Model file for the job. Use its own axes, mm. Face numbers are marked on the shaded views. A direction names the side the tool comes from. Round coordinates to 2 decimals unless told otherwise and drop trailing zeros. Write each loop counter-clockwise with the first axis right and the second up, starting at its lowest first coordinate (ties: lowest second). Pieces come first, ordered by that corner, then holes. Notation, with made-up numbers: (13.5, -36) - (52.5, -36) arc R18 ccw to (52.5, -19) - close; hole circle Ø9 at (0.25, 64.5). An arc over 180 degrees is marked (long way). Answer as a JSON object with one key per item and string values. Group by question number.
from build123d import *

# Parameters (mm, degrees)
SKETCH1_W           = 52
SKETCH1_H           = 50
BOSS_EXTRUDE1_DEPTH = 4
SKETCH2_R           = 1.75
SKETCH2_R_2         = 11
CUT_EXTRUDE1_DEPTH  = 37.290494623
SKETCH3_W           = 4
SKETCH3_H           = 50
BOSS_EXTRUDE3_DEPTH = 48
BOSS_EXTRUDE4_START = -50
SKETCH5_W           = 20
SKETCH5_H           = 10
BOSS_EXTRUDE4_DEPTH = 50
SKETCH7_W           = 20
SKETCH7_H           = 44
CUT_EXTRUDE2_DEPTH  = 10
CUT_EXTRUDE3_DEPTH  = 77.681158051
CUT_EXTRUDE5_DEPTH  = 78.672388917
CUT_EXTRUDE6_DEPTH  = 61.041652209
CUT_EXTRUDE7_DEPTH  = 64.285069329


with BuildPart() as part:
    # Sketch1 → Boss-Extrude1 (new body)
    with BuildSketch(Plane(origin=(0, 0, 0), x_dir=(1, 0, 0), z_dir=(0, 1, 0))):
        Rectangle(SKETCH1_W, SKETCH1_H)
    extrude(amount=BOSS_EXTRUDE1_DEPTH)

    # Sketch2 → Cut-Extrude1 (cut, through all)
    with BuildSketch(Plane(origin=(0, 4, 0), x_dir=(1, 0, 0), z_dir=(0, 1, 0))):
        with Locations(Location((19, 15.5, 0), (0, 0, 270))):
            Circle(SKETCH2_R)
        with Locations(Location((-12, -15.5, 0), (0, 0, 90))):
            Circle(SKETCH2_R)
        with Locations(Location((19, -15.5, 0), (0, 0, 270))):
            Circle(SKETCH2_R)
        with Locations(Location((-12, 15.5, 0), (0, 0, 90))):
            Circle(SKETCH2_R)
        with Locations(Location((3.5, 0, 0), (0, 0, 270))):
            Circle(SKETCH2_R_2)
    extrude(amount=-CUT_EXTRUDE1_DEPTH, mode=Mode.SUBTRACT)

    # Sketch3 → Boss-Extrude3 (add)
    with BuildSketch(Plane(origin=(0, 4, 0), x_dir=(1, 0, 0), z_dir=(0, 1, 0))):
        with Locations((-24, 0)):
            Rectangle(SKETCH3_W, SKETCH3_H)
    extrude(amount=BOSS_EXTRUDE3_DEPTH)

    # Sketch5 → Boss-Extrude4 (add)
    with BuildSketch(Plane.XY.offset(25).offset(BOSS_EXTRUDE4_START)):
        with Locations((-12, 9)):
            Rectangle(SKETCH5_W, SKETCH5_H)
    extrude(amount=BOSS_EXTRUDE4_DEPTH)

    # Sketch7 → Cut-Extrude2 (cut)
    with BuildSketch(Plane(origin=(0, 14, 0), x_dir=(1, 0, 0), z_dir=(0, 1, 0))):
        with Locations((-12, 0)):
            Rectangle(SKETCH7_W, SKETCH7_H)
    extrude(amount=-CUT_EXTRUDE2_DEPTH, mode=Mode.SUBTRACT)

    # Sketch8 → Cut-Extrude3 (cut, through all)
    with BuildSketch(Plane.XY.offset(25)):
        Polygon((-22, 14), (-2, 4), (-2, 14), align=None)
    extrude(amount=-CUT_EXTRUDE3_DEPTH, mode=Mode.SUBTRACT)

    # Sketch9 → Cut-Extrude5 (cut, through all)
    with BuildSketch(Plane.ZY.offset(26)):
        with BuildLine():
            Line((-13.75, 47.315114044), (-13.75, 8.684885956))
            ThreePointArc((-13.75, 8.684885956), (-15.5, 6.934885956), (-17.25, 8.684885956))
            Line((-17.25, 8.684885956), (-17.25, 47.315114044))
            ThreePointArc((-17.25, 47.315114044), (-15.5, 49.065114044), (-13.75, 47.315114044))
        make_face()
        with BuildLine():
            Line((17.25, 47.315114044), (17.25, 8.684885956))
            ThreePointArc((17.25, 8.684885956), (15.5, 6.934885956), (13.75, 8.684885956))
            Line((13.75, 8.684885956), (13.75, 47.315114044))
            ThreePointArc((13.75, 47.315114044), (15.5, 49.065114044), (17.25, 47.315114044))
        make_face()
    extrude(amount=-CUT_EXTRUDE5_DEPTH, mode=Mode.SUBTRACT)

    # Sketch11 → Cut-Extrude6 (cut, through all)
    with BuildSketch(Plane(origin=(0, 4, 0), x_dir=(1, 0, 0), z_dir=(0, 1, 0))):
        with BuildLine():
            Line((-16.2, 17.25), (-7.8, 17.25))
            ThreePointArc((-7.8, 17.25), (-6.05, 15.5), (-7.8, 13.75))
            Line((-7.8, 13.75), (-16.2, 13.75))
            ThreePointArc((-16.2, 13.75), (-17.95, 15.5), (-16.2, 17.25))
        make_face()
        with BuildLine():
            Line((-16.2, -17.25), (-7.8, -17.25))
            ThreePointArc((-7.8, -17.25), (-6.05, -15.5), (-7.8, -13.75))
            Line((-7.8, -13.75), (-16.2, -13.75))
            ThreePointArc((-16.2, -13.75), (-17.95, -15.5), (-16.2, -17.25))
        make_face()
        with BuildLine():
            Line((23.2, 13.75), (14.8, 13.75))
            ThreePointArc((14.8, 13.75), (13.05, 15.5), (14.8, 17.25))
            Line((14.8, 17.25), (23.2, 17.25))
            ThreePointArc((23.2, 17.25), (24.95, 15.5), (23.2, 13.75))
        make_face()
        with BuildLine():
            Line((23.2, -13.75), (14.8, -13.75))
            ThreePointArc((14.8, -13.75), (13.05, -15.5), (14.8, -17.25))
            Line((14.8, -17.25), (23.2, -17.25))
            ThreePointArc((23.2, -17.25), (24.95, -15.5), (23.2, -13.75))
        make_face()
    extrude(amount=-CUT_EXTRUDE6_DEPTH, mode=Mode.SUBTRACT)

    # Sketch12 → Cut-Extrude7 (cut, through all)
    with BuildSketch(Plane.XZ):
        with BuildLine():
            Line((3.5, -11), (-4.5, -11))
            ThreePointArc((-4.5, -11), (-15.5, 0), (-4.5, 11))
            Line((-4.5, 11), (3.5, 11))
            ThreePointArc((3.5, 11), (14.5, 0), (3.5, -11))
        make_face()
    extrude(amount=-CUT_EXTRUDE7_DEPTH, mode=Mode.SUBTRACT)


solid = part.part
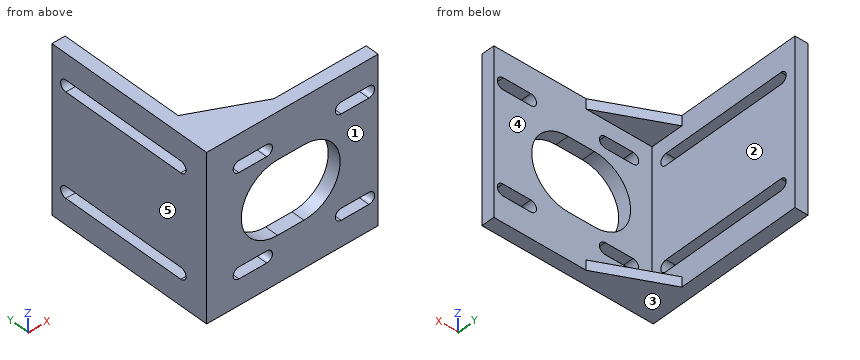
(1) Pull direction Z, two halves, no side cores. Call the marked faces 3, 4 and 5: pulls with the +Z half, pulls with the -Z half, needs draft (parallel to the pull), parting line crosses it, or undercut.
(2) Slice it at D-D (y = 5). Write the cut outline in (x, z).
(3) Slice it at B-B (y = 32). Write the cut outline in (x, z).
(4) Slice it at A-A (z = 0). Write the cut outline in (x, y).
(5) 3-axis set-ups, long thin cutter, end or side, ignore diameter. For the marked faces 1 and 2: which of +Z, -Z, +X, -X, +Y, -Y reach the whole face in a straight line?
(6) Slice it at C-C (z = 15.5). Write the cut outline in (x, y), then the cut area to 3 significant figures.
(7) Drill centre lines: line 1 (Z direction, x = -22.5, y = 7.5); line 2 (X direction, y = 6, z = 10); line 3 (Y direction, x = 22, z = -13.5). Where is each one in solid material? Low to high. Write a range as from..to.
(8) Flat gauge pins, fed straight in: pin 1 (5 mm diameter, centred on x = 16, z = 10, fed in from +Y); pin 2 (24 mm diameter, centred on y = 37.5, z = 1, fed in from +X). Where does each tip first touch, or does it go through?
Answer:
{
 "1": {"face 3": "pulls with the -Z half", "face 4": "undercut", "face 5": "needs draft"},
 "2": {"outline": "(-26, -25) - (-4, -25) - (-4, -22) - (-22, -22) - (-22, 22) - (-4, 22) - (-4, 25) - (-26, 25) - close"},
 "3": {"outline": "(-26, -25) - (-22, -25) - (-22, -17.25) - (-26, -17.25) - close; (-26, -13.75) - (-22, -13.75) - (-22, 13.75) - (-26, 13.75) - close; (-26, 17.25) - (-22, 17.25) - (-22, 25) - (-26, 25) - close"},
 "4": {"outline": "(-26, 0) - (-15.5, 0) - (-15.5, 4) - (-22, 4) - (-22, 52) - (-26, 52) - close; (14.5, 0) - (26, 0) - (26, 4) - (14.5, 4) - close"},
 "5": {"face 1": "+Z, -Z, +X, -X, -Y", "face 2": "+X, +Y"},
 "6": {"outline": "(-26, 0) - (-17.95, 0) - (-17.95, 4) - (-22, 4) - (-22, 6.93) - (-26, 6.93) - close; (-26, 49.07) - (-22, 49.07) - (-22, 52) - (-26, 52) - close; (-6.05, 0) - (13.05, 0) - (13.05, 4) - (-6.05, 4) - close; (24.95, 0) - (26, 0) - (26, 4) - (24.95, 4) - close", "area": "136 mm²"},
 "7": {"line 1": "-25..-16.79, -14.21..14.21, 16.79..25", "line 2": "-26..-22", "line 3": "0..4"},
 "8": {"pin 1": "y = 4", "pin 2": "x = -22"}
}
